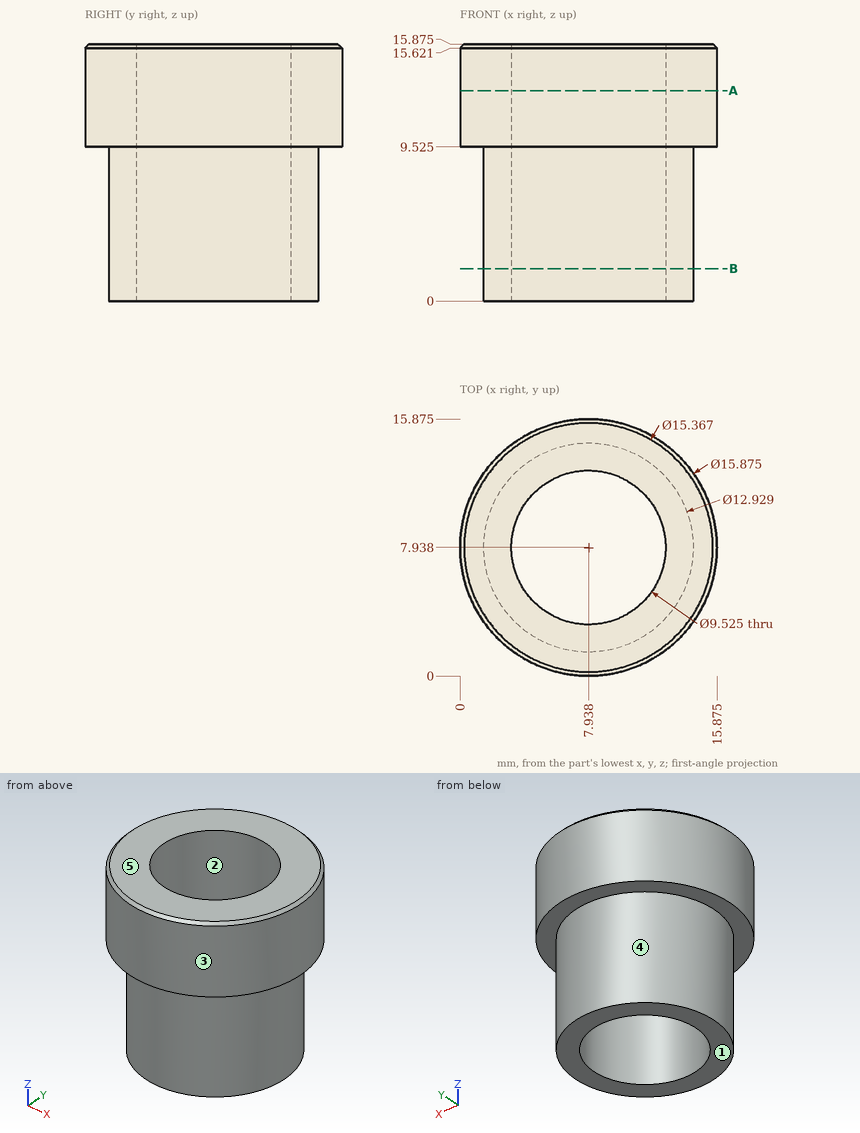
Input: dimensioned drawing with shaded views. Units: mm. Origin: part minimum x, y, z. A direction names the side the tool comes from. Give positions to 0.01 mm unless a question says otherwise; leave off trailing zeros. Write each loop counter-clockwise with the first axis right and the second up, starting at its lowest first coordinate (ties: lowest second). Pieces come first, ordered by that corner, then holes.
Q1. Section B-B, the plane z = 2. Output: boundary loops of the cut face in (x, y) (1 decimal).
Q2. Set-up query: the marked faces 4 and 5. Return all of +Z, -Z, +X, -X, +Y, -Y with unobstructed straight access to the full face (end or side cutting, diameter ignored); none if empty.
Q3. Pull-direction query (X, two-part tool) for the marked faces 1, 2 and 3; classes: pulls with the +X half, pulls with the -X half, needs draft (parallel to the pull), parting line crosses it, or undercut.
Q4. First-contact query: P1, Ø5, axis at x = 10, z = 2, coming from the -Y side; P2, Ø3, axis at y = 2, z = 11, coming from the -X side (1 decimal); P3, Ø1.5, axis at y = 2, z = 8, coming from the +X side (1 decimal); P4, Ø8, axis at x = 6, z = 11.5, coming from the +Y side (1 decimal). Flat tips, straight axial feed; report the tip coordinate or a pass-through.
Q5. Section A-A, the plane z = 13. Output: boundary loops of the cut face in (x, y) (1 decimal), plus the area to 3 significant figures.
Q6. Material intervals for probe 1 along Y at (x, z) = (8, 10.75) (1 decimal); probe 2 along X at (y, z) = (10.25, 14.5) (1 decimal), sorted ascending.
Filled in:
1. outline: circle Ø12.9 at (7.9, 7.9); hole circle Ø9.5 at (7.9, 7.9)
2. face 4: -Z
2. face 5: +Z, +X, -X, +Y, -Y
3. face 1: needs draft
3. face 2: undercut
3. face 3: parting line crosses it
4. P1: stops at y = 1.47
4. P2: stops at x = 1.4
4. P3: stops at x = 11.8
4. P4: stops at y = 15.9
5. outline: circle Ø15.9 at (7.9, 7.9); hole circle Ø9.5 at (7.9, 7.9)
5. area: 127 mm2
6. probe 1: y = 0 to 3.2, 12.7 to 15.9
6. probe 2: x = 0.3 to 3.8, 12.1 to 15.5
